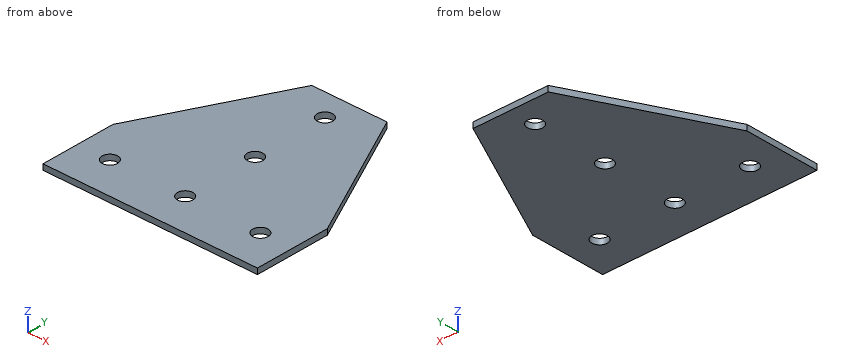
```python
from build123d import *

# Parameters (mm, degrees)
SKETCH_1_R        = 4.1
EXTRUDE_405_DEPTH = 1.5


with BuildPart() as part:
    # Эскиз1 → Extrude 405 (new, symmetric)
    with BuildSketch(Plane.XY):
        Polygon((-57, -20), (57, -20), (57, 20), (20, 94), (-20, 94), (-57, 20), align=None)
        Circle(SKETCH_1_R, mode=Mode.SUBTRACT)
        with Locations((-40, 0)):
            Circle(SKETCH_1_R, mode=Mode.SUBTRACT)
        with Locations((40, 0)):
            Circle(SKETCH_1_R, mode=Mode.SUBTRACT)
        with Locations((0, 40)):
            Circle(SKETCH_1_R, mode=Mode.SUBTRACT)
        with Locations((0, 80)):
            Circle(SKETCH_1_R, mode=Mode.SUBTRACT)
    extrude(amount=EXTRUDE_405_DEPTH, both=True)


solid = part.part
```
The model under review builds one solid part; all positions refer to its coordinate system, in mm. Round coordinates to 2 decimals unless told otherwise and drop trailing zeros. Loops run counter-clockwise (first coordinate to the right, second up) from the corner with the lowest first, then second, coordinate; pieces in that order, holes last. Notation, with made-up numbers: (41, 36.25) - (70, 36.25) arc R15 cw to (70, 54.25) - close; hole circle Ø2 at (-13, 19). An arc over 180 degrees is marked (long way). Use a Markdown table: item, result. Add a question column.
Q1. Add section B-B (y = 0). State the section outline as (x, z) points.
Q2. Add section D-D (x = 0). State the section outline as (y, z) points.
Q3. Add section C-C (z = -0.05). State the section outline as (x, y) points, plus the area to 3 significant figures.
Q4. Add section A-A (x = 40). State the section outline as (y, z) points.
Q5. For probe 1 along Y at (x, z) = (0, 0.85); probe 2 along X at (y, z) = (3.5, -0.4); probe 3 along Y at (x, z) = (38.5, 1.15), list the stretches that pass through material, from the lowest coordinate up.
Q6. Insertion check: pin 1 Ø7.5 at (x, y) = (0, 80) entering from +Z. The pin has a flat end and moves straight along its axis. Give the tip position at first contact, or say it passes through.
Worked answers:
| question | item | result |
|---|---|---|
| 1 | outline | (-57, -1.5) - (-44.1, -1.5) - (-44.1, 1.5) - (-57, 1.5) - close; (-35.9, -1.5) - (-4.1, -1.5) - (-4.1, 1.5) - (-35.9, 1.5) - close; (4.1, -1.5) - (35.9, -1.5) - (35.9, 1.5) - (4.1, 1.5) - close; (44.1, -1.5) - (57, -1.5) - (57, 1.5) - (44.1, 1.5) - close |
| 2 | outline | (-20, -1.5) - (-4.1, -1.5) - (-4.1, 1.5) - (-20, 1.5) - close; (4.1, -1.5) - (35.9, -1.5) - (35.9, 1.5) - (4.1, 1.5) - close; (44.1, -1.5) - (75.9, -1.5) - (75.9, 1.5) - (44.1, 1.5) - close; (84.1, -1.5) - (94, -1.5) - (94, 1.5) - (84.1, 1.5) - close |
| 3 | outline | (-57, -20) - (57, -20) - (57, 20) - (20, 94) - (-20, 94) - (-57, 20) - close; hole circle Ø8.2 at (-40, 0); hole circle Ø8.2 at (0, 0); hole circle Ø8.2 at (0, 40); hole circle Ø8.2 at (0, 80); hole circle Ø8.2 at (40, 0) |
| 3 | area | 9,990 mm² |
| 4 | outline | (-20, -1.5) - (-4.1, -1.5) - (-4.1, 1.5) - (-20, 1.5) - close; (4.1, -1.5) - (54, -1.5) - (54, 1.5) - (4.1, 1.5) - close |
| 5 | probe 1 | -20 to -4.1, 4.1 to 35.9, 44.1 to 75.9, 84.1 to 94 |
| 5 | probe 2 | -57 to -42.14, -37.86 to -2.14, 2.14 to 37.86, 42.14 to 57 |
| 5 | probe 3 | -20 to -3.82, 3.82 to 57 |
| 6 | pin 1 | through |
